Source: CAD feature listing. Evaluate the final solid. Frame: model axes, mm. A direction names the side the tool comes from. Coordinates: 2 decimals unless noted, no trailing zeros. Loops run counter-clockwise (first coordinate to the right, second up) from the corner with the lowest first, then second, coordinate; pieces in that order, holes last.
Item 1: Pull-direction query (Z, two-part tool) for faces 4 (the cylindrical face through (23.72, -94.65, -45.605)), 5 (the flat face through (-13, -185.4, -48)), 6 (the cylindrical face through (-49.61, 40.86, 4.17)), 7 (the cylindrical face through (47.01, -72.01, 14.8)); classes: +Z half, -Z half, draft (parallel to the pull), parting line (faces both ways), or undercut.
Item 2: Pin query (flat end, axial travel): pin 1 Ø5 at (y, z) = (-151.5, 14) entering from -X; pin 2 Ø1 at (x, y) = (37, 63) entering from -Z; pin 3 Ø12 at (y, z) = (46.5, 21.5) entering from +X. Return the tip coordinate at first contact, or that it passes through.
Item 3: Section query B-B, the plane z = -7. State how many separate pieces and enclosed holes the cut face has, then the cut area to 3 significant figures.
Item 4: Line query: probe 1 along Z at (x, y) = (0, 53.75); probe 2 along X at (y, z) = (-104, 0); probe 3 along Z at (x, y) = (-36, 0). Output: solid intervals per line, ascending.
Item 5: Section query C-C, the plane y = -103. Return the cut outline in (x, z).
Item 6: Section query A-A, the plane y = 53. Return the cut outline in (x, z), then the cut area to 3 significant figures.
Item 7: Reachability of faces 1 (the cylindrical face through (57.23, 34.51, 18.02)), 2 (the flat face through (8, 70, -49)), 3 (the flat face through (38, 125.4, -32)) from +Z, -Z, +X, -X, +Y, -Y: full face, straight path, thin tool, end or side. Return the list, or none.
```python
from build123d import *

# Parameters (mm, degrees)
F0_R      = 60
F1_DEPTH  = 70
F2_R      = 60
F3_DEPTH  = 70
F3_TAPER  = 7
F5_R      = 54.9341030365
F6_DEPTH  = 25.4
F7_R      = 47.9617586767
F8_DEPTH  = 205.994
F4_R      = 51.4050807368
F12_DEPTH = 50
F13_R     = 51.4050807368
F14_DEPTH = 25.4
F14_TAPER = -7
F15_R     = 53.9269190887
F16_DEPTH = 40
F16_TAPER = -7
F11_R     = 60
F17_DEPTH = 25.4
F17_TAPER = -3
F18_R     = 61.3311575938
F19_DEPTH = 30
F19_TAPER = -3
F20_R     = 46.550299856
F21_DEPTH = 374.396
F22_R     = 49.2833226897
F23_DEPTH = 359.918
F24_R     = 41.0727260018
F25_DEPTH = 101.854


with BuildPart() as f1:
    # F0 (on Front) → F1 (new body)
    with BuildSketch(Plane.XZ):
        Circle(F0_R)
    extrude(amount=-F1_DEPTH)

    # F2 (on face) → F3 (join)
    with BuildSketch(Plane.XZ):
        Circle(F2_R)
    extrude(amount=F3_DEPTH, taper=F3_TAPER)

    # F5 (on face) → F6 (cut)
    with BuildSketch(Plane(origin=(0, 70, 0), x_dir=(-1, 0, 0), z_dir=(0, 1, 0))):
        Circle(F5_R)
    extrude(amount=-F6_DEPTH, mode=Mode.SUBTRACT)

    # F7 (on face) → F8 (cut)
    with BuildSketch(Plane.XZ.offset(70)):
        Circle(F7_R)
    extrude(amount=-F8_DEPTH, mode=Mode.SUBTRACT)

    # F4 (on face) → F12 (join)
    with BuildSketch(Plane.XZ.offset(70)):
        Circle(F4_R)
    extrude(amount=F12_DEPTH)

    # F13 (on face) → F14 (join)
    with BuildSketch(Plane.XZ.offset(120)):
        Circle(F13_R)
    extrude(amount=F14_DEPTH, taper=F14_TAPER)

    # F15 (on face) → F16 (join)
    with BuildSketch(Plane.XZ.offset(145.4)):
        Circle(F15_R)
    extrude(amount=F16_DEPTH, taper=F16_TAPER)

    # F11 (on face) → F17 (join)
    with BuildSketch(Plane(origin=(0, 70, 0), x_dir=(-1, 0, 0), z_dir=(0, 1, 0))):
        Circle(F11_R)
    extrude(amount=F17_DEPTH, taper=F17_TAPER)

    # F18 (on face) → F19 (join)
    with BuildSketch(Plane(origin=(0, 95.4, 0), x_dir=(-1, 0, 0), z_dir=(0, 1, 0))):
        Circle(F18_R)
    extrude(amount=F19_DEPTH, taper=F19_TAPER)

    # F20 (on face) → F21 (cut)
    with BuildSketch(Plane.XZ.offset(185.4)):
        Circle(F20_R)
    extrude(amount=-F21_DEPTH, mode=Mode.SUBTRACT)

    # F22 (on face) → F23 (cut)
    with BuildSketch(Plane.XZ.offset(185.4)):
        Circle(F22_R)
    extrude(amount=-F23_DEPTH, mode=Mode.SUBTRACT)

    # F24 (on Right) → F25 (cut)
    with BuildSketch(Plane.YZ):
        Circle(F24_R)
    extrude(amount=-F25_DEPTH, mode=Mode.SUBTRACT)


solid = f1.part
```
Verdict:
1. face 4: parting line
1. face 5: draft
1. face 6: undercut
1. face 7: undercut
2. pin 1: stops at x = -53.54
2. pin 2: stops at z = -47.62
2. pin 3: stops at x = 57.96
3. separate pieces: 3
3. enclosed holes: 0
3. area: 3,690 mm2
4. probe 1: z = -60 to -54.93, 54.93 to 60
4. probe 2: x = -51.41 to -49.28, 49.28 to 51.41
4. probe 3: z = -48 to -41.07, 41.07 to 48
5. outline: circle Ø102.81 at (0, 0); hole circle Ø98.57 at (0, 0)
6. outline: circle Ø120 at (0, 0); hole circle Ø109.87 at (0, 0)
6. area: 1,830 mm2
7. face 1: -Y
7. face 2: none
7. face 3: +Z, -Z, +X, -X, +Y
